```python
from build123d import *

# Parameters (mm, degrees)
F0_W     = 27.1898097297
F0_H     = 16.2868271582
F1_DEPTH = 25


with BuildPart() as f1:
    # F0 (on Top) → F1 (new body)
    with BuildSketch(Plane.XY):
        with BuildLine():
            ThreePointArc((-296.8951798975, -48.7195744038), (-292.5017816153, -59.3261761216), (-281.8951798975, -63.7195744038))
            Line((-281.8951798975, -63.7195744038), (-142.0774715642, -63.7195744038))
            ThreePointArc((-142.0774715642, -63.7195744038), (-131.5723208853, -59.4266659422), (-127.0801902383, -49.0051489655))
            ThreePointArc((-127.0801902383, -49.0051489655), (-162.3644421178, -13.7181785166), (-127.0801902383, 21.5687919322))
            ThreePointArc((-127.0801902383, 21.5687919322), (-131.5723208853, 31.990308909), (-142.0774715642, 36.2832173705))
            Line((-142.0774715642, 36.2832173705), (-281.8951798975, 36.2832173705))
            ThreePointArc((-281.8951798975, 36.2832173705), (-292.5017816153, 31.8898190883), (-296.8951798975, 21.2832173705))
            Line((-296.8951798975, 21.2832173705), (-296.8951798975, 21.2820385972))
            ThreePointArc((-296.8951798975, 21.2820385972), (-261.8949627837, -13.7181785166), (-296.8951798975, -48.7183956304))
            Line((-296.8951798975, -48.7183956304), (-296.8951798975, -48.7195744038))
        make_face()
        Polygon((-296.8951798975, -21.1222618818), (-296.8951798975, -22.4110819399), (-274.3184268475, -22.4110819399), (-274.3184268475, -5.8417902328), (-296.8951798975, -5.8417902328), align=None)
        with Locations((-140.672376429, -13.9852038119)):
            Rectangle(F0_W, F0_H)
        with BuildLine():
            Line((-296.8951798975, -35.9437018633), (-296.8951798975, -48.7183956304))
            ThreePointArc((-296.8951798975, -48.7183956304), (-261.8949627837, -13.7181785166), (-296.8951798975, 21.2820385972))
            Line((-296.8951798975, 21.2820385972), (-296.8951798975, 0))
            Line((-296.8951798975, 0), (-296.8951798975, -5.8417902328))
            Line((-296.8951798975, -5.8417902328), (-274.3184268475, -5.8417902328))
            Line((-274.3184268475, -5.8417902328), (-274.3184268475, -22.4110819399))
            Line((-274.3184268475, -22.4110819399), (-296.8951798975, -22.4110819399))
            Line((-296.8951798975, -22.4110819399), (-296.8951798975, -35.9437018633))
        make_face()
        with BuildLine():
            ThreePointArc((-127.0801902383, 21.5687919322), (-162.3644421178, -13.7181785166), (-127.0801902383, -49.0051489655))
            ThreePointArc((-127.0801902383, -49.0051489655), (-127.0781512481, -48.8623681549), (-127.0774715642, -48.7195744038))
            Line((-127.0774715642, -48.7195744038), (-127.0774715642, -36.2968184054))
            Line((-127.0774715642, -36.2968184054), (-127.0774715642, -22.4110819399))
            Line((-127.0774715642, -22.4110819399), (-127.0774715642, -22.128617391))
            Line((-127.0774715642, -22.128617391), (-154.2672812939, -22.128617391))
            Line((-154.2672812939, -22.128617391), (-154.2672812939, -5.8417902328))
            Line((-154.2672812939, -5.8417902328), (-127.0774715642, -5.8417902328))
            Line((-127.0774715642, -5.8417902328), (-127.0774715642, 21.2832173705))
            ThreePointArc((-127.0774715642, 21.2832173705), (-127.0781512481, 21.4260111217), (-127.0801902383, 21.5687919322))
        make_face()
    extrude(amount=F1_DEPTH)


solid = f1.part
```
Geometry check sheet. Reference: the model listing, model coordinates, mm. Give positions to 0.01 mm unless a question says otherwise; leave off trailing zeros. Write each loop counter-clockwise with the first axis right and the second up, starting at its lowest first coordinate (ties: lowest second). Pieces come first, ordered by that corner, then holes. Notation, with made-up numbers: (28, 33) -> (38, 33) arc R18 cw to (38, 47) -> close; hole circle Ø6 at (42, 83.5). An arc over 180 degrees is marked (long way). One line per question, with ' | ' between items.
Item 1: Scan lines: line 1 along X through (y, z) = (-56.5, 11); line 2 along X through (y, z) = (-52.5, 1.5). Record each from-to range of solid material in increasing order.
Determined:
line 1: -294.72 to -129.25 | line 2: -296.41 to -127.56
Item 2: Depth check by flat-ended pin: pin 1 (4 mm diameter, centred on y = -52, z = 10.5, fed in from +X); pin 2 (8 mm diameter, centred on y = 25.5, z = 16.5, fed in from -X). Enter the tip coordinate at first touch or a pass-through.
Determined:
pin 1: x = -127.13 | pin 2: x = -296.89
Item 3: Sectioned sample at A-A, the plane y = -55.5. Record the boundary of the cut face in (x, z), plus the area to 3 significant figures.
Determined:
outline: (-295.28, 0) -> (-128.7, 0) -> (-128.7, 25) -> (-295.28, 25) -> close | area: 4,160 mm^2
